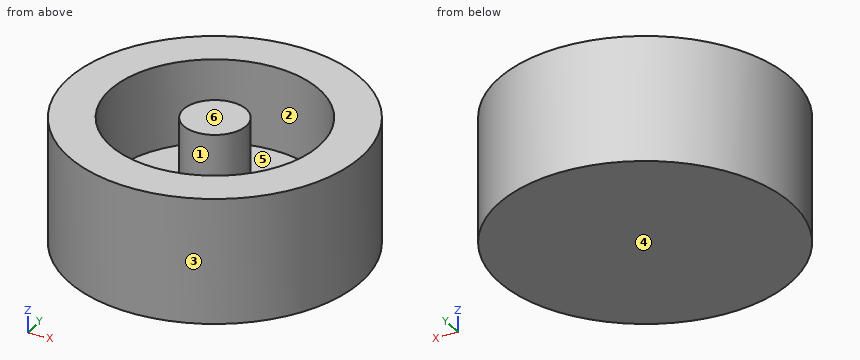
from build123d import *

# Parameters (mm, degrees)
CROQUIS1_R              = 3.5
SALIENTE_EXTRUIR1_DEPTH = 3
CROQUIS2_R              = 2.5
CORTAR_EXTRUIR1_DEPTH   = 2
CROQUIS3_R              = 0.75
SALIENTE_EXTRUIR2_DEPTH = 2


with BuildPart() as part:
    # Croquis1 → Saliente-Extruir1 (new body)
    with BuildSketch(Plane.XY):
        Circle(CROQUIS1_R)
    extrude(amount=SALIENTE_EXTRUIR1_DEPTH)

    # Croquis2 → Cortar-Extruir1 (cut)
    with BuildSketch(Plane.XY.offset(3)):
        Circle(CROQUIS2_R)
    extrude(amount=-CORTAR_EXTRUIR1_DEPTH, mode=Mode.SUBTRACT)

    # Croquis3 → Saliente-Extruir2 (add)
    with BuildSketch(Plane.XY.offset(1)):
        Circle(CROQUIS3_R)
    extrude(amount=SALIENTE_EXTRUIR2_DEPTH)


solid = part.part
Could you check a few things on this model? Use its own coordinates, in mm. Face numbers are marked on the shaded views. A direction names the side the tool comes from. Coordinates: 2 decimals unless noted, no trailing zeros. Write each loop counter-clockwise with the first axis right and the second up, starting at its lowest first coordinate (ties: lowest second). Pieces come first, ordered by that corner, then holes. Notation, with made-up numbers: M 12.25,62 L 59.25,62 A24 cw 59.25,83 Z; hole C 11,20.25 d5. An arc over 180 degrees is marked long. One line per question, with ' | ' between items.
1) For the marked faces 5 and 6, which set-ups out of +Z, -Z, +X, -X, +Y, -Y let a thin tool reach every point of the face, with its end or its side?
Checks:
face 5: +Z | face 6: +Z, +X, -X, +Y, -Y
2) If we mould it in two halves opening along Y, with no side actions, what happens to the marked faces 1, 2, 3 and 4? For each: released by +Y, released by -Y, zero draft, split by the parting line, or undercut.
Checks:
face 1: undercut | face 2: undercut | face 3: split by the parting line | face 4: zero draft
3) I need wall thicknesses on probe 1 along Y at (x, z) = (0, 2.5); probe 2 along Y at (x, z) = (-0.5, 2.45); probe 3 along Z at (x, y) = (1, -1). Which ranges of each line are inside material? Lowest first, please. Write a range as [from, to].
Checks:
probe 1: [-3.5, -2.5], [-0.75, 0.75], [2.5, 3.5] | probe 2: [-3.46, -2.45], [-0.56, 0.56], [2.45, 3.46] | probe 3: [0, 1]
4) For pin 1 Ø1.5 at (x, z) = (-1, 2) entering from +Y, with a flat end and sliding along its axis, tell me the tip position at first contact or that it passes through.
Checks:
pin 1: y = 3.49
5) Imagine slicing it at C-C, the plane z = 1.7. Write out the boundary of the cut face in (x, y).
Checks:
outline: C 0,0 d7; C 0,0 d1.5; hole C 0,0 d5
6) Imagine slicing it at A-A, the plane y = 0. Write out the boundary of the cut face in (x, z), and give its area (3 significant figures).
Checks:
outline: M -3.5,0 L 3.5,0 L 3.5,3 L 2.5,3 L 2.5,1 L 0.75,1 L 0.75,3 L -0.75,3 L -0.75,1 L -2.5,1 L -2.5,3 L -3.5,3 Z | area: 14.0 mm²
7) Imagine slicing it at D-D, the plane x = 1.5. Write out the boundary of the cut face in (y, z).
Checks:
outline: M -3.16,0 L 3.16,0 L 3.16,3 L 2,3 L 2,1 L -2,1 L -2,3 L -3.16,3 Z
